Read the model definition and answer for the solid it produces. Units are mm, in the model's axes. A direction names the side the tool comes from. Give positions to 0.01 mm unless a question says otherwise; leave off trailing zeros. Order: outer loops, then holes, each group sorted by start corner. A loop starts at its lowest first (then second) coordinate and runs counter-clockwise, first axis right, second up. Notation, with made-up numbers: (-39.5, 78) - (-26.5, 78) arc R18 cw to (-26.5, 86) - close; hole circle Ø10 at (29, -8). An arc over 180 degrees is marked (long way). Write item = value, one per line.
```python
from build123d import *

# Parameters (mm, degrees)
BOSS_EXTRUDE1_DEPTH  = 70
SKETCH2_R            = 2.25
SKETCH2_W            = 41.8
SKETCH2_H            = 21.1
CUT_EXTRUDE1_DEPTH   = 6
LPATTERN1_COUNT      = 4
LPATTERN1_PITCH      = 14
LPATTERN1_COUNT_DIR2 = 2
LPATTERN1_PITCH_DIR2 = 55
SKETCH4_W            = 36.2
SKETCH4_H            = 8
BOSS_EXTRUDE2_DEPTH  = 50
SKETCH5_W            = 36.2
SKETCH5_H            = 8
BOSS_EXTRUDE3_DEPTH  = 50
SKETCH6_W            = 172.2
SKETCH6_H            = 8
BOSS_EXTRUDE4_DEPTH  = 20.2
SKETCH7_W            = 172.2
SKETCH7_H            = 36.2
BOSS_EXTRUDE5_DEPTH  = 8
SKETCH8_R            = 4
CUT_EXTRUDE2_DEPTH   = 147.830991279
LPATTERN2_COUNT      = 6
LPATTERN2_PITCH      = 24.6
SKETCH9_R            = 4
CUT_EXTRUDE3_DEPTH   = 151.720038482


with BuildPart() as part:
    # Sketch1 → Boss-Extrude1 (new body)
    with BuildSketch(Plane.XY):
        Polygon((0, 26.7), (0, 0), (72.2, 0), (72.2, 61.7), (66.2, 61.7), (66.2, 26.7), (55, 26.7), (55, 13.5), (61, 13.5), (61, 18.7), (66.2, 18.7), (66.2, 6), (6, 6), (6, 18.7), (11.2, 18.7), (11.2, 13.5), (17.2, 13.5), (17.2, 26.7), align=None)
    extrude(amount=BOSS_EXTRUDE1_DEPTH)

    # Sketch2 → Cut-Extrude1 (cut)
    with BuildSketch(Plane.ZY.offset(-66.2)):
        with Locations(Location((10.25, 49.13, 0), (0, 0, 270))):
            Circle(SKETCH2_R)
        with Locations(Location((10.25, 39.13, 0), (0, 0, 270))):
            Circle(SKETCH2_R)
        with Locations(Location((59.75, 49.13, 0), (0, 0, 270))):
            Circle(SKETCH2_R)
        with Locations(Location((59.75, 39.13, 0), (0, 0, 270))):
            Circle(SKETCH2_R)
        with Locations((35, 44.13)):
            Rectangle(SKETCH2_W, SKETCH2_H)
    extrude(amount=-CUT_EXTRUDE1_DEPTH, mode=Mode.SUBTRACT)

    # Sketch3 → Cut-Revolve1 (revolve, cut)
    with BuildSketch(Plane.XZ.offset(-18.7)):
        with BuildLine():
            Line((61.1, 56), (66.1, 56))
            ThreePointArc((66.1, 56), (63.6, 58.5), (61.1, 56))
        make_face()
    cut_revolve1 = revolve(axis=Axis((61.1, 18.7, 56), (1, 0, 0)), mode=Mode.SUBTRACT)

    # LPattern1: Cut-Revolve1 4 × 2
    with Locations(*[(-j * LPATTERN1_PITCH_DIR2, 0, -i * LPATTERN1_PITCH) for i in range(LPATTERN1_COUNT) for j in range(LPATTERN1_COUNT_DIR2) if (i, j) != (0, 0)]):
        add(cut_revolve1, mode=Mode.SUBTRACT)

    # Sketch4 → Boss-Extrude2 (add)
    with BuildSketch(Plane(origin=(72.2, 0, 0), x_dir=(0, 0, -1), z_dir=(1, 0, 0))):
        with Locations((-35, 4)):
            Rectangle(SKETCH4_W, SKETCH4_H)
    extrude(amount=BOSS_EXTRUDE2_DEPTH)

    # Sketch5 → Boss-Extrude3 (add)
    with BuildSketch(Plane.ZY):
        with Locations((35, 4)):
            Rectangle(SKETCH5_W, SKETCH5_H)
    extrude(amount=BOSS_EXTRUDE3_DEPTH)

    # Sketch6 → Boss-Extrude4 (add)
    with BuildSketch(Plane.XZ):
        with Locations((36.1, 49.1)):
            Rectangle(SKETCH6_W, SKETCH6_H)
        with Locations((36.1, 20.9)):
            Rectangle(SKETCH6_W, SKETCH6_H)
    extrude(amount=BOSS_EXTRUDE4_DEPTH)

    # Sketch7 → Boss-Extrude5 (add)
    with BuildSketch(Plane.XZ.offset(20.2)):
        with Locations((36.1, 35)):
            Rectangle(SKETCH7_W, SKETCH7_H)
    extrude(amount=BOSS_EXTRUDE5_DEPTH)

    # Sketch8 → Cut-Extrude2 (cut, through all)
    with BuildSketch(Plane.XY.offset(53.1)):
        with Locations((-25.4, -10.1)):
            Circle(SKETCH8_R)
    cut_extrude2 = extrude(amount=-CUT_EXTRUDE2_DEPTH, mode=Mode.SUBTRACT)

    # LPattern2: Cut-Extrude2 ×6
    with Locations(*[(i * LPATTERN2_PITCH, 0, 0) for i in range(1, LPATTERN2_COUNT)]):
        add(cut_extrude2, mode=Mode.SUBTRACT)

    # Sketch9 → Cut-Extrude3 (cut, through all)
    with BuildSketch(Plane(origin=(0, 8, 0), x_dir=(1, 0, 0), z_dir=(0, 1, 0))):
        with Locations(Location((-37.7, -35, 0), (0, 0, 180))):
            Circle(SKETCH9_R)
        with Locations(Location((-13.1, -35, 0), (0, 0, 180))):
            Circle(SKETCH9_R)
    cut_extrude3 = extrude(amount=-CUT_EXTRUDE3_DEPTH, mode=Mode.SUBTRACT)

    # Mirror1: Cut-Extrude3 across plane
    add(cut_extrude3.mirror(Plane.ZY.offset(-36.1)), mode=Mode.SUBTRACT)


solid = part.part
```
1. For faces 1 (the face through (9, 26.7, 35)), 2 (the face through (69, 44, 55.9)), 3 (the face through (58, 13.5, 35)), 4 (the face through (55, 20, 35)), determine the directions among +Z, -Z, +X, -X, +Y, -Y from which every point of the face is accessible in a straight line to the end or side of a thin tool.
Recorded:
face_1 = +Z, -Z, -X, +Y
face_2 = +X, -X
face_3 = +Z, -Z
face_4 = +Z, -Z, +Y
2. Section C-C (y = 39.13) is taken. Determine the outline of the cut face in (x, z), and give its area (3 significant figures).
Recorded:
outline = (66.2, 0) - (72.2, 0) - (72.2, 8) - (66.2, 8) - close; (66.2, 12.5) - (72.2, 12.5) - (72.2, 14.1) - (66.2, 14.1) - close; (66.2, 55.9) - (72.2, 55.9) - (72.2, 57.5) - (66.2, 57.5) - close; (66.2, 62) - (72.2, 62) - (72.2, 70) - (66.2, 70) - close
area = 115 mm^2
3. Determine the mould class of faces 5 (the face through (-21.585, -8.899, 20.956)), 6 (the face through (66.2, 33, 35)), 7 (the face through (39, 4, 70)) for opening direction X: +X half, -X half, draft (parallel to the pull), parting line (faces both ways), or undercut.
Recorded:
face_5 = undercut
face_6 = -X half
face_7 = draft
4. Section B-B (x = 23.8) is taken. Determine the outline of the cut face in (y, z).
Recorded:
outline = (-28.2, 16.9) - (-14.1, 16.9) - (-14.1, 24.9) - (-20.2, 24.9) - (-20.2, 45.1) - (-14.1, 45.1) - (-14.1, 53.1) - (-28.2, 53.1) - close; (-6.1, 16.9) - (0, 16.9) - (0, 0) - (6, 0) - (6, 70) - (0, 70) - (0, 53.1) - (-6.1, 53.1) - (-6.1, 45.1) - (0, 45.1) - (0, 24.9) - (-6.1, 24.9) - close
5. Straight lines are drawn through the part: L1, parallel to Y at x = 97.6, z = 50; L2, parallel to Y at x = -19, z = 30; L3, parallel to Z at x = -25, y = -17. For each, find the intervals that lie inside material, in ascending order. Write a range as [from, to].
Recorded:
L1 = [-28.2, -14.1], [-6.1, 8]
L2 = [-28.2, -20.2], [0, 8]
L3 = [16.9, 24.9], [45.1, 53.1]
6. Section A-A (z = 47.5) is taken. Count the separate pieces of the cut face and the enclosed holes in it, and give its area (3 significant figures).
Recorded:
separate_pieces = 2
enclosed_holes = 6
area = 6,360 mm^2
7. Section D-D (y = 11) is taken. Determine the outline of the cut face in (x, z).
Recorded:
outline = (0, 0) - (6, 0) - (6, 70) - (0, 70) - close; (66.2, 0) - (72.2, 0) - (72.2, 70) - (66.2, 70) - close
8. Flat-ended cylindrical pins translate along their axes: pin 1 (4 mm diameter, centred on y = 15.5, z = 46, fed in from -X); pin 2 (5 mm diameter, centred on y = 49.13, z = 59.75, fed in from -X); pin 3 (6 mm diameter, centred on x = 74.5, y = -15, fed in from +Z). Find the tip coordinate at first contact, or state that the pin passes through.
Recorded:
pin_1 = 0
pin_2 = 66.2
pin_3 = 53.1
